Input: dimensioned drawing with shaded views. Units: mm. Origin: part minimum x, y, z. Round coordinates to 2 decimals unless told otherwise and drop trailing zeros. Order: outer loops, then holes, each group sorted by start corner. A loop starts at its lowest first (then second) coordinate and runs counter-clockwise, first axis right, second up. Notation, with made-up numbers: M -3.75,-13 L 51.25,-13 A27 cw 51.25,11 Z; hole C -12,-20 d10. An arc over 180 degrees is marked long. Use one line per item in the form item = value. Start each with the question number.
Q1. Material intervals for probe 1 along Y at (x, z) = (31, 2.55) (1 decimal); probe 2 along Y at (x, z) = (42, 2.3) (1 decimal); probe 3 along X at (y, z) = (25.5, 1.1) (1 decimal), sorted ascending.
Q2. Section C-C (y = 41.5). Return the cut outline in (x, z) (1 decimal).
Q3. Section B-B (z = 1.45). Return the cut outline in (x, y), plus the area to 3 significant figures.
Q4. Contact query for flat-ended pins moving along their axis: pin 1 (1.4 mm diameter, centred on x = 40.5, z = 2, fed in from -Y); pin 2 (6 mm diameter, centred on x = 50, y = 45, fed in from -Z). Output: stop coordinate, or through.
Q5. Section A-A (x = 43.5). Return the cut outline in (y, z).
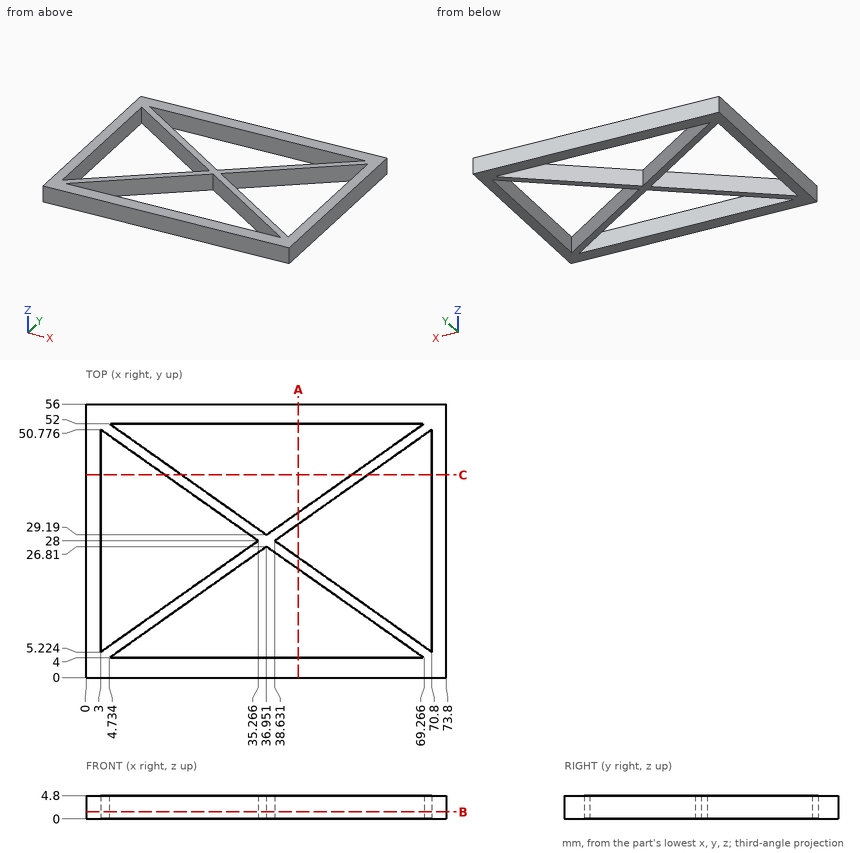
Results list:
q1.probe_1 = 0 to 4, 22.6 to 25, 31 to 33.4, 52 to 56
q1.probe_2 = 0 to 4, 23.2 to 25.6, 30.4 to 32.8, 52 to 56
q1.probe_3 = 0 to 3, 31.7 to 35.1, 38.8 to 42.2, 70.8 to 73.8
q2.outline = M 0,0 L 3,0 L 3,4.8 L 0,4.8 Z; M 16.1,0 L 19.6,0 L 19.6,4.8 L 16.1,4.8 Z; M 54.4,0 L 57.7,0 L 57.7,4.8 L 54.4,4.8 Z; M 70.8,0 L 73.8,0 L 73.8,4.8 L 70.8,4.8 Z
q3.outline = M 0,0 L 73.8,0 L 73.8,56 L 0,56 Z; hole M 3,5.22 L 35.27,28 L 3,50.78 Z; hole M 4.73,4 L 69.27,4 L 36.95,26.81 Z; hole M 4.73,52 L 36.95,29.19 L 69.27,52 Z; hole M 38.63,28 L 70.8,5.22 L 70.8,50.78 Z
q3.area = 1,190 mm2
q4.pin_1 = 0
q4.pin_2 = through
q5.outline = M 0,0 L 4,0 L 4,4.8 L 0,4.8 Z; M 22.19,0 L 24.55,0 L 24.55,4.8 L 22.19,4.8 Z; M 31.45,0 L 33.81,0 L 33.81,4.8 L 31.45,4.8 Z; M 52,0 L 56,0 L 56,4.8 L 52,4.8 Z
